Autodesk Inventor part; units mm, degrees
ref_plane "YZ Plane" through (0, 0, 0) normal (1, 0, 0) x (0, 1, 0)
ref_plane "XZ Plane" through (0, 0, 0) normal (0, 1, 0) x (-1, 0, 0)
ref_plane "XY Plane" through (0, 0, 0) normal (0, 0, 1) x (1, 0, 0)
sketch "Sketch1" plane through (0, 0, 0) normal (0, 0, 1) x (1, 0, 0)
  line L0 (-25, 15.75) -> (25, 15.75)
  line L1 (25, 15.75) -> (25, -15.75)
  line L2 (25, -15.75) -> (20, -15.75)
  line L3 (20, -15.75) -> (20, -14.75)
  line L4 (20, -14.75) -> (-18, -14.75)
  line L5 (-18, -14.75) -> (-18, 3.75)
  line L6 (-18, 3.75) -> (-25, 3.75)
  line L7 (-25, 3.75) -> (-25, 15.75)
  line L8 (-35, 0) -> (35, 0) construction
  line L9 (0, -22.05) -> (0, 22.05) construction
  point P0 (0, 0)
  dimension "d0" = 50
  dimension "d1" = 31.5
  dimension "d2" = 1
  dimension "d3" = 7
  dimension "d5" = 5
  dimension "d24" = 12
  dimension "d25" = 19.5
extrude "Extrusion1" add sketch "Sketch1" along normal mid plane 40
sketch "Sketch2" plane through (-25, 15.75, 20) normal (0, 1, 0) x (1, 0, 0)
  line L0 (45, 40) -> (45, 0) construction
  line L1 (7, 0) -> (45, 0) construction
  line L2 (7, 40) -> (7, 0) construction
  line L3 (45, 40) -> (7, 40) construction
  line L4 (0, 40) -> (50, 40)
  line L5 (25, 40) -> (25, 0)
  line L6 (50, 0) -> (0, 0)
  point P0 (25, 20)
  point P1 (25, 20)
  dimension "d23" = 18
  dimension "d26" = 38
hole "Hole1" at (0, 15.75, 0) direction (0, -1, 0) diameter 10.5 end through all counterbore diameter 18 counterbore depth 10
chamfer "Chamfer1" distance 2 angle 45 6 edges at (-25, 15.75, 0) (0, 15.75, 20) (0, 15.75, -20) (25, 15.75, 0) (25, 0, 20) (25, 0, -20)
chamfer "Chamfer2" distance 4 angle 45 2 edges at (-25, 8.75, 20) (-25, 8.75, -20)
chamfer "Chamfer3" distance 0.5 angle 45 1 edges at (0, -14.75, -5.25)
chamfer "Chamfer4" distance 0.5 angle 45 1 edges at (0, 15.75, -9)
properties part number "VTC1-001"
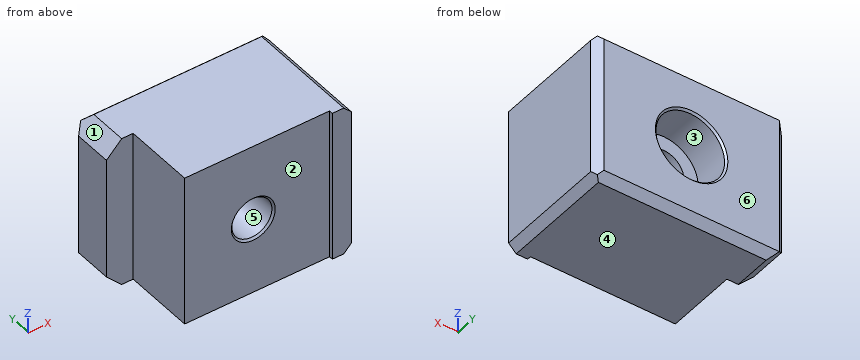
Check sheet for the modelled part. Datum: model origin and axes. Units: mm. Face numbers are marked on the shaded views. A direction names the side the tool comes from. Coordinates: 2 decimals unless noted, no trailing zeros. Write each loop counter-clockwise with the first axis right and the second up, starting at its lowest first coordinate (ties: lowest second). Pieces come first, ordered by that corner, then holes. Notation, with made-up numbers: M 86,67.25 L 137,67.25 A18 cw 137,83.25 Z; hole C 84.5,-26.75 d5. An arc over 180 degrees is marked long. Use one line per item in the form item = value.
Item 1: Sectioned sample at C-C, the plane y = -8. Record the cut outline in (x, z).
Answer below:
outline = M -18,-20 L 23,-20 L 25,-18 L 25,18 L 23,20 L -18,20 Z; hole C 0,0 d10.5
Item 2: Gauge pin test, flat ends, axial feed: pin 1 Ø1.1 at (y, z) = (-15, -1.5) entering from -X; pin 2 Ø8 at (x, z) = (-5.5, -6.5) entering from -Y; pin 3 Ø5 at (y, z) = (2.5, 13) entering from -X; pin 4 Ø16 at (x, z) = (0, 0) entering from +Y. Record the tip position at first contact, or that the pin passes through.
Answer below:
pin_1 = -18
pin_2 = -14.75
pin_3 = -25
pin_4 = 5.75
Item 3: Material ranges on L1, parallel to X at y = -0.5, z = 0; L2, parallel to X at y = 10, z = 0; L3, parallel to Z at x = 0, y = -11.5, recorded low to high. Write a range as from..to.
Answer below:
L1 = -18..-5.25, 5.25..25
L2 = -25..-9, 9..25
L3 = -20..-5.25, 5.25..20
Item 4: Release check for a two-part mould opening along Z. For the marked faces 3, 4, 5 and 6 record: pulls with the +Z half, pulls with the -Z half, needs draft (parallel to the pull), parting line crosses it, or undercut.
Answer below:
face_3 = undercut
face_4 = pulls with the -Z half
face_5 = undercut
face_6 = needs draft
Item 5: Sectioned sample at B-B, the plane x = 0. Record the cut outline in (y, z), and give its area (3 significant figures).
Answer below:
outline = M -14.75,-20 L 13.75,-20 L 15.75,-18 L 15.75,-9.5 L 15.25,-9 L 5.75,-9 L 5.75,-5.25 L -14.25,-5.25 L -14.75,-5.75 Z; M -14.75,5.75 L -14.25,5.25 L 5.75,5.25 L 5.75,9 L 15.25,9 L 15.75,9.5 L 15.75,18 L 13.75,20 L -14.75,20 Z
area = 820 mm^2
Item 6: Sectioned sample at A-A, the plane z = 0. Record the cut outline in (x, y), and give its area (3 significant figures).
Answer below:
outline = M -25,3.75 L -18,3.75 L -18,-14.75 L -5.75,-14.75 L -5.25,-14.25 L -5.25,5.75 L -9,5.75 L -9,15.25 L -9.5,15.75 L -23,15.75 L -25,13.75 Z; M 5.25,-14.25 L 5.75,-14.75 L 20,-14.75 L 20,-15.75 L 25,-15.75 L 25,13.75 L 23,15.75 L 9.5,15.75 L 9,15.25 L 9,5.75 L 5.25,5.75 Z
area = 1,000 mm^2
Item 7: Sectioned sample at D-D, the plane x = 19. Record the cut outline in (y, z), and give its area (3 significant figures).
Answer below:
outline = M -14.75,-20 L 13.75,-20 L 15.75,-18 L 15.75,18 L 13.75,20 L -14.75,20 Z
area = 1,220 mm^2
Item 8: Set-up check for the marked faces 1 and 2: record each of +Z, -Z, +X, -X, +Y, -Y from which the full face is reachable in a straight line by a thin tool's end or side.
Answer below:
face_1 = +Z, -X, +Y, -Y
face_2 = +Z, -Z, -X, -Y
